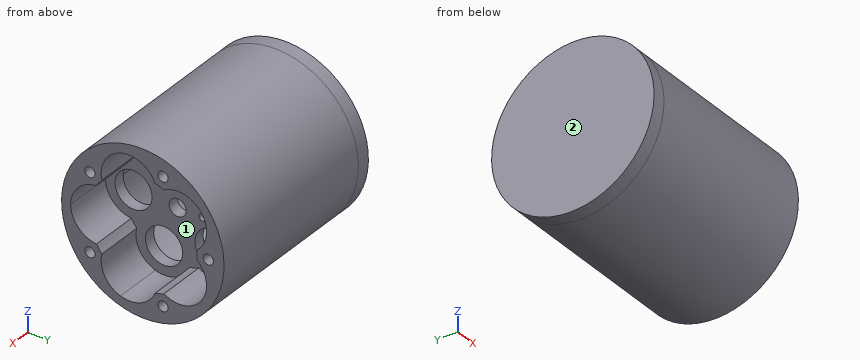
from build123d import *

# Parameters (mm, degrees)
SKETCH1_R                = 16
SKETCH1_R_2              = 4.125
BOSS_EXTRUDE1_DEPTH      = 2.5
SKETCH2_R                = 18
SKETCH2_R_2              = 16
BOSS_EXTRUDE2_DEPTH      = 10.5
BOSS_EXTRUDE2_DEPTH_BACK = 30
SKETCH3_R                = 18
BOSS_EXTRUDE3_DEPTH      = 3
SKETCH4_R                = 1.89865
CUT_EXTRUDE1_DEPTH       = 3
BOSS_EXTRUDE4_DEPTH      = 31
SKETCH6_R                = 0.75
CUT_EXTRUDE2_DEPTH       = 3
BOSS_EXTRUDE5_DEPTH      = 10.5
SKETCH8_R                = 1.1303
CUT_EXTRUDE3_DEPTH       = 23


with BuildPart() as part:
    # Sketch1 → Boss-Extrude1 (new body)
    with BuildSketch(Plane(origin=(0, 0, 0), x_dir=(0, 0, -1), z_dir=(1, 0, 0))):
        Circle(SKETCH1_R)
        with Locations((-5.75, 7.914196043)):
            Circle(SKETCH1_R_2, mode=Mode.SUBTRACT)
        with Locations((5.75, 7.914196043)):
            Circle(SKETCH1_R_2, mode=Mode.SUBTRACT)
        with Locations((9.303695435, -3.022953895)):
            Circle(SKETCH1_R_2, mode=Mode.SUBTRACT)
        with Locations((0, -9.782484296)):
            Circle(SKETCH1_R_2, mode=Mode.SUBTRACT)
        with Locations((-9.303695435, -3.022953895)):
            Circle(SKETCH1_R_2, mode=Mode.SUBTRACT)
    extrude(amount=BOSS_EXTRUDE1_DEPTH)

    # Sketch2 → Boss-Extrude2 (add, two sides)
    with BuildSketch(Plane(origin=(2.5, 0, 0), x_dir=(0, 0, -1), z_dir=(1, 0, 0))) as boss_extrude2_sk:
        Circle(SKETCH2_R)
        Circle(SKETCH2_R_2, mode=Mode.SUBTRACT)
    extrude(amount=BOSS_EXTRUDE2_DEPTH)
    extrude(boss_extrude2_sk.sketch, amount=-BOSS_EXTRUDE2_DEPTH_BACK)

    # Sketch3 → Boss-Extrude3 (add)
    with BuildSketch(Plane.ZY.offset(27.5)):
        Circle(SKETCH3_R)
    extrude(amount=BOSS_EXTRUDE3_DEPTH)

    # Sketch4 → Cut-Extrude1 (cut)
    with BuildSketch(Plane(origin=(2.5, 0, 0), x_dir=(0, 0, -1), z_dir=(1, 0, 0))):
        Circle(SKETCH4_R)
    extrude(amount=-CUT_EXTRUDE1_DEPTH, mode=Mode.SUBTRACT)

    # Sketch5 → Boss-Extrude4 (add)
    with BuildSketch(Plane(origin=(2.5, 0, 0), x_dir=(0, 0, -1), z_dir=(1, 0, 0))):
        Polygon((-0.75, -15), (-0.5, -14.75), (0.5, -14.75), (0.75, -15), (0.75, -16.25), (-0.75, -16.25), align=None)
    extrude(amount=-BOSS_EXTRUDE4_DEPTH)

    # Sketch6 → Cut-Extrude2 (cut)
    with BuildSketch(Plane(origin=(2.5, 0, 0), x_dir=(0, 0, -1), z_dir=(1, 0, 0))):
        with Locations((0, 5.5)):
            Circle(SKETCH6_R)
    extrude(amount=-CUT_EXTRUDE2_DEPTH, mode=Mode.SUBTRACT)

    # Sketch7 → Boss-Extrude5 (add)
    with BuildSketch(Plane(origin=(2.5, 0, 0), x_dir=(0, 0, -1), z_dir=(1, 0, 0))):
        with BuildLine():
            ThreePointArc((-9.404564054, 12.944271897), (-5.021788452, 14.088919475), (-1.025538841, 11.956097611))
            ThreePointArc((-1.025538841, 11.956097611), (0, 12), (1.025538841, 11.956097611))
            ThreePointArc((1.025538841, 11.956097611), (5.021788614, 14.088919494), (9.404564318, 12.944271706))
            ThreePointArc((9.404564318, 12.944271706), (1.63e-07, 16), (-9.404564054, 12.944271897))
        make_face()
        with BuildLine():
            ThreePointArc((-11.054015612, 4.669982746), (-11.847540705, 9.12972016), (-9.404564054, 12.944271897))
            ThreePointArc((-9.404564054, 12.944271897), (-15.216904236, 4.944271986), (-15.216904316, -4.944271739))
            ThreePointArc((-15.216904316, -4.944271739), (-14.951176606, -0.422288989), (-11.687833473, 2.719291951))
            ThreePointArc((-11.687833473, 2.719291951), (-11.412678196, 3.708203932), (-11.054015612, 4.669982746))
        make_face()
        with BuildLine():
            ThreePointArc((-7.857296202, -9.069889547), (-12.343971357, -8.446442057), (-15.216904316, -4.944271739))
            ThreePointArc((-15.216904316, -4.944271739), (-9.40456411, -12.944271857), (0, -16))
            ThreePointArc((0, -16), (-4.218546896, -14.349908473), (-6.1979395, -10.27548276))
            ThreePointArc((-6.1979395, -10.27548276), (-7.053423028, -9.708203932), (-7.857296202, -9.069889547))
        make_face()
        with BuildLine():
            ThreePointArc((6.1979395, -10.27548276), (4.218546896, -14.349908473), (0, -16))
            ThreePointArc((0, -16), (9.404563995, -12.944271941), (15.216904229, -4.944272009))
            ThreePointArc((15.216904229, -4.944272009), (12.343971234, -8.446442126), (7.857296202, -9.069889547))
            ThreePointArc((7.857296202, -9.069889547), (7.053423028, -9.708203932), (6.1979395, -10.27548276))
        make_face()
        with BuildLine():
            ThreePointArc((16, 0), (14.256104466, 7.263847841), (9.404564318, 12.944271706))
            ThreePointArc((9.404564318, 12.944271706), (11.847540737, 9.12972), (11.054015612, 4.669982746))
            ThreePointArc((11.054015612, 4.669982746), (11.412678196, 3.708203932), (11.687833473, 2.719291951))
            ThreePointArc((11.687833473, 2.719291951), (14.951176666, -0.422289118), (15.216904229, -4.944272009))
            ThreePointArc((15.216904229, -4.944272009), (15.803013441, -2.502951492), (16, 0))
        make_face()
    extrude(amount=BOSS_EXTRUDE5_DEPTH)

    # Sketch8 → Cut-Extrude3 (cut)
    with BuildSketch(Plane(origin=(13, 0, 0), x_dir=(0, 0, -1), z_dir=(1, 0, 0))):
        with Locations((0, 14.5)):
            Circle(SKETCH8_R)
        with Locations((13.790319486, 4.480746418)):
            Circle(SKETCH8_R)
        with Locations((8.522886158, -11.730746418)):
            Circle(SKETCH8_R)
        with Locations((-8.522886158, -11.730746418)):
            Circle(SKETCH8_R)
        with Locations((-13.790319486, 4.480746418)):
            Circle(SKETCH8_R)
    extrude(amount=-CUT_EXTRUDE3_DEPTH, mode=Mode.SUBTRACT)


solid = part.part
Check sheet for the modelled part. Datum: model origin and axes. Units: mm. Face numbers are marked on the shaded views. Round coordinates to 2 decimals unless told otherwise and drop trailing zeros. Order: outer loops, then holes, each group sorted by start corner. A loop starts at its lowest first (then second) coordinate and runs counter-clockwise, first axis right, second up.
Q1. Cross-section at A-A, the plane x = -23. Enter the section's corners in (y, z), plus the area to 3 significant figures.
Filled sheet:
outline: circle Ø36 at (0, 0); hole (-15.98, -0.75) arc R16 ccw (long way) to (-15.98, 0.75) - (-15, 0.75) - (-14.75, 0.5) - (-14.75, -0.5) - (-15, -0.75) - close
area: 215 mm2
Q2. Cross-section at D-D, the plane z = -10.5. Enter the section's corners in (x, y), plus the area to 3 significant figures.
Filled sheet:
outline: (-30.5, -14.62) - (13, -14.62) - (13, -9.12) - (2.5, -9.12) - (2.5, -6.97) - (0, -6.97) - (0, -12.07) - (-27.5, -12.07) - (-27.5, 12.07) - (0, 12.07) - (0, 0.92) - (2.5, 0.92) - (2.5, 11.93) - (13, 11.93) - (13, 14.62) - (-30.5, 14.62) - close
area: 367 mm2
Q3. Cross-section at C-C, the plane x = 7. Enter the section's corners in (y, z), plus the area to 3 significant figures.
Filled sheet:
outline: circle Ø36 at (0, 0); hole circle Ø2.26 at (-11.73, -8.52); hole circle Ø2.26 at (-11.73, 8.52); hole (-10.28, -6.2) arc R12 ccw to (-9.07, -7.86) arc R6.22 ccw to (2.72, -11.69) arc R12 ccw to (4.67, -11.05) arc R6.22 ccw to (11.96, -1.03) arc R12 ccw to (11.96, 1.03) arc R6.22 ccw to (4.67, 11.05) arc R12 ccw to (2.72, 11.69) arc R6.22 ccw to (-9.07, 7.86) arc R12 ccw to (-10.28, 6.2) arc R6.22 ccw to start; hole circle Ø2.26 at (4.48, -13.79); hole circle Ø2.26 at (4.48, 13.79); hole circle Ø2.26 at (14.5, 0)
area: 345 mm2
Q4. Scan lines: L1, parallel to X at y = 10, z = 1; L2, parallel to Y at x = -26.5, z = 0.5; L3, parallel to Y at x = 1.5, z = 8. Record each from-to range of solid material in increasing order.
Filled sheet:
L1: x = -30.5 to -27.5, 0 to 2.5
L2: y = -17.99 to -14.75, 15.99 to 17.99
L3: y = -16.12 to -12.73, -10.73 to -6.94, 0.89 to 4.46, 11.37 to 16.12
Q5. Cross-section at B-B, the plane y = 7. Enter the section's corners in (x, z), plus the area to 3 significant figures.
Filled sheet:
outline: (-30.5, -16.58) - (13, -16.58) - (13, -11.9) - (2.5, -11.9) - (2.5, -9.77) - (0, -9.77) - (0, -14.39) - (-27.5, -14.39) - (-27.5, 14.39) - (0, 14.39) - (0, 9.77) - (2.5, 9.77) - (2.5, 11.9) - (13, 11.9) - (13, 16.58) - (-30.5, 16.58) - close; (0, -1.73) - (2.5, -1.73) - (2.5, 1.73) - (0, 1.73) - close
area: 361 mm2
Q6. Depth check by flat-ended pin: P1, Ø3.5, axis at y = 0, z = 0, coming from the +X side; P2, Ø9.5, axis at y = -1.5, z = 0, coming from the +X side; P3, Ø6, axis at x = -10, y = 10.5, coming from the +Z side. Enter the tip coordinate at first touch or a pass-through.
Filled sheet:
P1: stops at x = -27.5
P2: stops at x = 2.5
P3: stops at z = 16.36
Q7. Draft check along Y on the marked faces 1 and 2. Enter one of: pulls with the +Y half, pulls with the -Y half, needs draft (parallel to the pull), parting line crosses it, or undercut.
Filled sheet:
face 1: undercut
face 2: needs draft
